from build123d import *
from OCP.BRepFilletAPI import BRepFilletAPI_MakeChamfer

# Parameters (mm, degrees)
SKETCH1_W           = 40
SKETCH1_H           = 28.8
BOSS_EXTRUDE1_DEPTH = 12
CHAMFER2_SIZE       = 8
CHAMFER2_SIZE2      = 16
SKETCH10_W          = 14
SKETCH10_H          = 18.8
CUT_EXTRUDE7_DEPTH  = 7
SKETCH11_W          = 40
SKETCH11_H          = 3
CUT_EXTRUDE8_DEPTH  = 8
CHAMFER3_SIZE       = 8
CHAMFER3_SIZE2      = 10
CUT_EXTRUDE9_REACH  = 39.06
SKETCH13_R          = 1.65
CUT_EXTRUDE10_DEPTH = 30.957302949
CUT_EXTRUDE2_DEPTH  = 6
CUT_EXTRUDE3_DEPTH  = 38.05995143
SKETCH2_R           = 1.65
CUT_EXTRUDE1_DEPTH  = 38.05995143
CUT_EXTRUDE4_DEPTH  = 10
CUT_EXTRUDE5_DEPTH  = 6
CUT_EXTRUDE6_DEPTH  = 29.744390757
CHAMFER4_SIZE       = 3
CHAMFER4_SIZE_2     = 5
CHAMFER5_SIZE       = 3
CHAMFER5_SIZE_2     = 5
CHAMFER6_SIZE2      = 7
CHAMFER6_SIZE       = 3.5
CHAMFER7_SIZE2      = 7
CHAMFER7_SIZE       = 3.5


# Some blends are built 0.0001 mm under size
with BuildPart() as part:
    # Sketch1 → Boss-Extrude1 (new body)
    with BuildSketch(Plane.XY):
        with Locations((0, 14.4)):
            Rectangle(SKETCH1_W, SKETCH1_H)
    extrude(amount=BOSS_EXTRUDE1_DEPTH)

    # Chamfer2
    chamfer2_edges = [part.edges().sort_by_distance(p)[0] for p in [
        (0, 28.8, 12),
    ]]
    chamfer2_side = [part.faces().sort_by_distance(p)[0] for p in [
        (0, 28.8, 6),
    ]]
    chamfer(chamfer2_edges, length=CHAMFER2_SIZE, length2=CHAMFER2_SIZE2, reference=chamfer2_side[0])

    # Sketch10 → Cut-Extrude7 (cut)
    with BuildSketch(Plane.XY.offset(12)):
        with Locations((-13, 19.4)):
            Rectangle(SKETCH10_W, SKETCH10_H)
        with Locations((13, 19.4)):
            Rectangle(SKETCH10_W, SKETCH10_H)
    extrude(amount=-CUT_EXTRUDE7_DEPTH, mode=Mode.SUBTRACT)

    # Sketch11 → Cut-Extrude8 (cut)
    with BuildSketch(Plane.XY.offset(12)):
        with Locations((0, 1.5)):
            Rectangle(SKETCH11_W, SKETCH11_H)
    extrude(amount=-CUT_EXTRUDE8_DEPTH, mode=Mode.SUBTRACT)

    # Chamfer3: one chamfer whose edges measure the first distance from different faces: ONE call of the kernel's chamfer builder (chamfer() names one face for all edges)
    chamfer3_edges_1 = [part.edges().sort_by_distance(p)[0] for p in [
        (-20, 6.5, 12),
    ]]
    chamfer3_side_1 = [part.faces().sort_by_distance(p)[0] for p in [
        (-20, 12.483950617, 4.012345679),
    ]]
    chamfer3_edges_2 = [part.edges().sort_by_distance(p)[0] for p in [
        (20, 6.5, 12),
    ]]
    chamfer3_side_2 = [part.faces().sort_by_distance(p)[0] for p in [
        (20, 12.483950617, 4.012345679),
    ]]
    chamfer3 = BRepFilletAPI_MakeChamfer(part.part.solid().wrapped)
    for e in chamfer3_edges_1:
        chamfer3.Add(CHAMFER3_SIZE, CHAMFER3_SIZE2, e.wrapped, chamfer3_side_1[0].wrapped)  # the first distance lies on this face
    for e in chamfer3_edges_2:
        chamfer3.Add(CHAMFER3_SIZE, CHAMFER3_SIZE2, e.wrapped, chamfer3_side_2[0].wrapped)  # the first distance lies on this face
    add(Compound.cast(chamfer3.Shape()), mode=Mode.REPLACE)

    # Cut-Extrude9: up to this face of the body (flat: up to its plane)
    cut_extrude9_end = Plane(part.part.faces().sort_by_distance((-10.56840796, 10, 7.890547264))[0])
    # Sketch12 → Cut-Extrude9 (cut, up to the picked face)
    with BuildSketch(Plane(origin=(0, 28.8, 0), x_dir=(1, 0, 0), z_dir=(0, 1, 0)), mode=Mode.PRIVATE) as cut_extrude9_sk1:
        with BuildLine():
            Line((-4.25, -8), (-4.25, -12))
            Line((-4.25, -12), (-10.75, -12))
            Line((-10.75, -12), (-10.75, -8))
            ThreePointArc((-10.75, -8), (-7.5, -4.75), (-4.25, -8))
        make_face()
    cut_extrude9_tool1 = split(extrude(cut_extrude9_sk1.sketch, amount=-CUT_EXTRUDE9_REACH, mode=Mode.PRIVATE), bisect_by=cut_extrude9_end, keep=Keep.BOTH, mode=Mode.PRIVATE)
    cut_extrude9 = cut_extrude9_tool1.solids().sort_by(Axis((-7.5, 28.8, 8.683577), (0, -1, 0)))[0]
    add(cut_extrude9, mode=Mode.SUBTRACT)

    # Sketch13 → Cut-Extrude10 (cut, through all)
    with BuildSketch(Plane(origin=(0, 10, 0), x_dir=(1, 0, 0), z_dir=(0, 1, 0))):
        with Locations(Location((-7.5, -8, 0), (0, 0, 180))):
            Circle(SKETCH13_R)
    cut_extrude10 = extrude(amount=-CUT_EXTRUDE10_DEPTH, mode=Mode.SUBTRACT)

    # Sketch3 → Cut-Extrude2 (cut)
    with BuildSketch(Plane.XZ):
        with BuildLine():
            Line((-5, 8), (-5, 12))
            Line((-5, 12), (5, 12))
            Line((5, 12), (5, 8))
            ThreePointArc((5, 8), (0, 3), (-5, 8))
        make_face()
    extrude(amount=-CUT_EXTRUDE2_DEPTH, mode=Mode.SUBTRACT)

    # Sketch4 → Cut-Extrude3 (cut, through all)
    with BuildSketch(Plane.XY.offset(12)):
        with BuildLine():
            Line((-3, 20.8), (-3, 28.8))
            Line((-3, 28.8), (3, 28.8))
            Line((3, 28.8), (3, 20.8))
            ThreePointArc((3, 20.8), (0, 17.8), (-3, 20.8))
        make_face()
    extrude(amount=-CUT_EXTRUDE3_DEPTH, mode=Mode.SUBTRACT)

    # Sketch2 → Cut-Extrude1 (cut, through all)
    with BuildSketch(Plane.XY.offset(12)):
        with Locations((-12.5, 2.8)):
            Circle(SKETCH2_R)
        with Locations((12.5, 2.8)):
            Circle(SKETCH2_R)
        with Locations((12.5, 25.8)):
            Circle(SKETCH2_R)
        with Locations((-12.5, 25.8)):
            Circle(SKETCH2_R)
    extrude(amount=-CUT_EXTRUDE1_DEPTH, mode=Mode.SUBTRACT)

    # Sketch5 → Cut-Extrude4 (cut)
    with BuildSketch(Plane.XY.offset(12)):
        Polygon((-13.803959833, 29.341475319), (-11.196040167, 29.341475319), (-9.151368439, 25.8), (-10.825684219, 22.9), (-14.174315781, 22.9), (-15.848631561, 25.8), align=None)
        Polygon((11.196040167, 29.341475319), (13.803959833, 29.341475319), (15.848631561, 25.8), (14.174315781, 22.9), (10.825684219, 22.9), (9.151368439, 25.8), align=None)
        Polygon((-9.151368439, 2.8), (-10.825684219, 5.7), (-14.174315781, 5.7), (-15.848631561, 2.8), (-14.174315781, -0.1), (-10.825684219, -0.1), align=None)
        Polygon((15.848631561, 2.8), (14.174315781, 5.7), (10.825684219, 5.7), (9.151368439, 2.8), (10.825684219, -0.1), (14.174315781, -0.1), align=None)
    extrude(amount=-CUT_EXTRUDE4_DEPTH, mode=Mode.SUBTRACT)

    # Sketch6 → Cut-Extrude5 (cut)
    with BuildSketch(Plane.XZ.offset(-6)):
        Polygon((-2.9, 12), (2.9, 12), (2.9, 6.325684219), (0, 4.651368439), (-2.9, 6.325684219), align=None)
    extrude(amount=-CUT_EXTRUDE5_DEPTH, mode=Mode.SUBTRACT)

    # Sketch7 → Cut-Extrude6 (cut, through all)
    with BuildSketch(Plane.XZ.offset(-12)):
        with BuildLine():
            Line((-1.5, 8.687386354), (-1.5, 12))
            Line((-1.5, 12), (1.5, 12))
            Line((1.5, 12), (1.5, 8.687386354))
            ThreePointArc((1.5, 8.687386354), (0, 6.35), (-1.5, 8.687386354))
        make_face()
    extrude(amount=-CUT_EXTRUDE6_DEPTH, mode=Mode.SUBTRACT)

    # Mirror1: Cut-Extrude9, Cut-Extrude10 across plane
    add(cut_extrude9.mirror(Plane(origin=(0, 0, 0), x_dir=(0, 0, 1), z_dir=(1, 0, 0))), mode=Mode.SUBTRACT)
    add(cut_extrude10.mirror(Plane(origin=(0, 0, 0), x_dir=(0, 0, 1), z_dir=(1, 0, 0))), mode=Mode.SUBTRACT)

    # Chamfer4
    # the kernel refuses this chamfer: 5, 3 mm, written as the material it takes off along each edge
    with BuildSketch(Plane(origin=(20, 28.8, -12.931305486), x_dir=(0.05518620705976579, -0.9984760801092616, 0), z_dir=(0, 0, 1))) as chamfer4_piece_1:
        Polygon((CHAMFER4_SIZE * 0.998476080109, -CHAMFER4_SIZE * 0.0551862070598), (-CHAMFER4_SIZE_2 * 0.0551862070598, -CHAMFER4_SIZE_2 * 0.998476080109), (0, 0), align=None)
    extrude(amount=29.862610972, mode=Mode.SUBTRACT)

    # Chamfer5
    # the kernel refuses this chamfer: 5, 3 mm, written as the material it takes off along each edge
    with BuildSketch(Plane(origin=(-20, 28.8, -12.931305486), x_dir=(-0.05518620705976579, -0.9984760801092616, 0), z_dir=(0, 0, 1))) as chamfer5_piece_1:
        Polygon((CHAMFER5_SIZE * 0.998476080109, CHAMFER5_SIZE * 0.0551862070598), (-CHAMFER5_SIZE_2 * 0.0551862070598, CHAMFER5_SIZE_2 * 0.998476080109), (0, 0), align=None)
    extrude(amount=29.862610972, mode=Mode.SUBTRACT)

    # Chamfer6
    chamfer6_edges = [part.edges().sort_by_distance(p)[0] for p in [
        (-3, 28.8, 2),
    ]]
    chamfer6_side = [part.faces().sort_by_distance(p)[0] for p in [
        (-3, 28.73, 2),
    ]]
    chamfer(chamfer6_edges, length=CHAMFER6_SIZE - 0.0001, length2=CHAMFER6_SIZE2 - 0.0001, reference=chamfer6_side[0])  # a hair under: the kernel refuses the full size

    # Chamfer7
    chamfer7_edges = [part.edges().sort_by_distance(p)[0] for p in [
        (3, 28.8, 2),
    ]]
    chamfer7_side = [part.faces().sort_by_distance(p)[0] for p in [
        (3, 28.73, 2),
    ]]
    chamfer(chamfer7_edges, length=CHAMFER7_SIZE - 0.0001, length2=CHAMFER7_SIZE2 - 0.0001, reference=chamfer7_side[0])  # a hair under: the kernel refuses the full size


solid = part.part
Check sheet for the modelled part. Datum: model origin and axes. Units: mm. A direction names the side the tool comes from. Round coordinates to 2 decimals unless told otherwise and drop trailing zeros. Loops run counter-clockwise (first coordinate to the right, second up) from the corner with the lowest first, then second, coordinate; pieces in that order, holes last.
1. Scan lines: probe 1 along Y at (x, z) = (12.5, 1.15); probe 2 along X at (y, z) = (27.25, 2.5); probe 3 along X at (y, z) = (3.5, 1.25). Record each from-to range of solid material in increasing order.
2. Mould release check, pull along Z, two halves, no side actions. Record for faces 1 (the cylindrical face through (-7.52, 18.77, 4.75)), 2 (the cylindrical face through (-6.284, 6.549, 9.115)), 3 (the flat face through (2.9, 9, 9)): released by +Z, released by -Z, zero draft, split by the parting line, or undercut.
3. Sectioned sample at A-A on x = 12.5. Record the boundary of the cut face in (y, z).
4. Sectioned sample at D-D on y = 16. Record the boundary of the cut face in (x, z), and give its area (3 significant figures).
5. Gauge pin test, flat ends, axial feed: pin 1 Ø3 at (y, z) = (10.5, 8.5) entering from -X; pin 2 Ø1.7 at (x, z) = (12.5, 6) entering from -Y; pin 3 Ø3 at (y, z) = (20, 7.5) entering from +X. Record the tip position at first contact, or that the pin passes through.
6. Set-up check for faces 4 (the flat face through (-14, 17, 5)), 5 (the flat face through (-2.2, 6, 5.6)), 6 (the cylindrical face through (4.735, 16.558, 6.292)), 7 (the flat face through (-20, 13, 2)), 8 (the flat face through (-9.97, 1.38, 3.01)): record each of +Z, -Z, +X, -X, +Y, -Y from which the full face is reachable in a straight line by a thin tool's end or side.
7. Sectioned sample at B-B on y = 9. Record the boundary of the cut face in (x, z).
8. Sectioned sample at C-C on z = 1.5. Record the boundary of the cut face in (x, y).
Recorded:
1. probe 1: y = 0 to 1.15, 4.45 to 24.15, 27.45 to 28.8
1. probe 2: x = -17.58 to -15.01, -9.99 to -6.9, 6.9 to 9.99, 15.01 to 17.58
1. probe 3: x = -20 to -13.99, -11.01 to 11.01, 13.99 to 20
2. face 1: released by +Z
2. face 2: undercut
2. face 3: zero draft
3. outline: (0, 0) - (1.15, 0) - (1.15, 2) - (0, 2) - close; (4.45, 0) - (24.15, 0) - (24.15, 2) - (22.9, 2) - (22.9, 5) - (10, 5) - (10, 10) - (5.7, 10) - (5.7, 2) - (4.45, 2) - close; (27.45, 0) - (28.8, 0) - (28.8, 2) - (27.45, 2) - close
4. outline: (-20, 0) - (20, 0) - (20, 4) - (18.75, 5) - (8.75, 5) arc R3.25 cw to (6.25, 5) - (6, 5) - (6, 5.12) arc R3.25 cw to (4.25, 8) - (4.25, 10.4) - (1.5, 10.4) - (1.5, 8.69) arc R1.65 cw (long way) to (-1.5, 8.69) - (-1.5, 10.4) - (-4.25, 10.4) - (-4.25, 8) arc R3.25 cw to (-6, 5.12) - (-6, 5) - (-6.25, 5) arc R3.25 cw to (-8.75, 5) - (-18.75, 5) - (-20, 4) - close
4. area: 235 mm2
5. pin 1: stops at x = -16.14
5. pin 2: stops at y = 5.7
5. pin 3: stops at x = 4.94
6. face 4: +Z, -X, +Y
6. face 5: +Z, -Y
6. face 6: +Z, +X, +Y
6. face 7: +Z, -Z, -X, +Y, -Y
6. face 8: +Z
7. outline: (-20, 0) - (20, 0) - (20, 4) - (10, 12) - (2.9, 12) - (2.9, 6.33) - (0, 4.65) - (-2.9, 6.33) - (-2.9, 12) - (-10, 12) - (-20, 4) - close; hole circle Ø3.3 at (-7.5, 8); hole circle Ø3.3 at (7.5, 8)
8. outline: (-20, 0) - (20, 0) - (20, 25.8) - (15, 28.8) - (10, 28.8) - (3, 25.3) - (3, 20.8) arc R3 cw to (-3, 20.8) - (-3, 25.3) - (-10, 28.8) - (-15, 28.8) - (-20, 25.8) - close; hole circle Ø3.3 at (-12.5, 2.8); hole circle Ø3.3 at (-12.5, 25.8); hole circle Ø3.3 at (12.5, 2.8); hole circle Ø3.3 at (12.5, 25.8)
